from build123d import *

# Parameters (mm, degrees)
SKETCH1_W                  = 75
SKETCH1_H                  = 75
BOSS_EXTRUDE1_DEPTH        = 60
SKETCH2_R                  = 5
CUT_EXTRUDE1_DEPTH         = 20
FILLET1_R                  = 3
CUT_EXTRUDE2_DEPTH         = 5
FILLET2_R                  = 5
FILLET2_OF_MIRROR1_R       = 5
MIRROR2_START              = -7.071067908
MIRROR2_DEPTH              = 14.142135816
SKETCH4_W                  = 25
SKETCH4_H                  = 20
CUT_EXTRUDE3_DEPTH         = 55
FILLET3_R                  = 5
CUT_EXTRUDE4_DEPTH         = 81.078087059
CUT_EXTRUDE4_DEPTH_BACK    = 81.078087059
SKETCH5_R                  = 7.5
SKETCH7_R                  = 15
CUT_EXTRUDE5_DEPTH         = 15
SKETCH8_R                  = 4.5
CUT_EXTRUDE6_DEPTH         = 11
M5_TAPPED_HOLE1_AT_2_COUNT = 2
M5_TAPPED_HOLE1_AT_2_PITCH = 36
M8_TAPPED_HOLE1_D          = 6.8
M8_TAPPED_HOLE1_DEPTH      = 19.75
M8_TAPPED_HOLE1_TIP        = 2.042926105
F_8_0MM_DOWEL_HOLE1_D      = 8


# Read off the part's stored shape, not the designer's step: Mirror2
with BuildPart() as part:
    # Sketch1 → Boss-Extrude1 (new, symmetric)
    with BuildSketch(Plane.XY):
        Rectangle(SKETCH1_W, SKETCH1_H)
    extrude(amount=BOSS_EXTRUDE1_DEPTH, both=True)

    # Sketch2 → Cut-Extrude1 (cut)
    with BuildSketch(Plane(origin=(0, 37.5, 0), x_dir=(1, 0, 0), z_dir=(0, 1, 0))):
        with Locations(Location((0, 0, 0), (0, 0, 270))):
            Circle(SKETCH2_R)
    extrude(amount=-CUT_EXTRUDE1_DEPTH, mode=Mode.SUBTRACT)

    # Fillet1
    fillet1_edges = [part.edges().sort_by_distance(p)[0] for p in [
        (-37.5, 37.5, 0),
        (37.5, 37.5, 0),
    ]]
    fillet(fillet1_edges, radius=FILLET1_R)

    # Sketch3 → Cut-Extrude2 (cut, symmetric)
    with BuildSketch(Plane.XY.offset(-25)):
        Polygon((-37.5, 27.5), (-27.5, 37.5), (-37.5, 37.5), align=None)
    cut_extrude2 = extrude(amount=CUT_EXTRUDE2_DEPTH, both=True, mode=Mode.SUBTRACT)

    # Fillet2
    fillet2_edges = [part.edges().sort_by_distance(p)[0] for p in [
        (-32.5, 32.5, -30),
        (-32.5, 32.5, -20),
    ]]
    fillet(fillet2_edges, radius=FILLET2_R - 0.0001)  # a hair under: the kernel refuses the full size

    # Mirror1: Cut-Extrude2 across plane
    add(cut_extrude2.mirror(Plane.XY), mode=Mode.SUBTRACT)

    # Fillet2 of Mirror1
    fillet2_of_mirror1_edges = [part.edges().sort_by_distance(p)[0] for p in [
        (-32.5, 32.5, 30),
        (-32.5, 32.5, 20),
    ]]
    fillet(fillet2_of_mirror1_edges, radius=FILLET2_OF_MIRROR1_R - 0.0001)  # a hair under: the kernel refuses the full size

    # Mirror2 outline → Mirror2 (cut)
    with BuildSketch(Plane(origin=(0, 0, 0), x_dir=(0.707106781186546, 0.707106781186549, 0), z_dir=(0.707106781186549, -0.707106781186546, 0)).offset(MIRROR2_START)):
        with BuildLine():
            ThreePointArc((50.961940783, 30.000000002), (45.961940781, 25), (50.961940783, 19.999999998))
            Line((50.961940783, 19.999999998), (53, 20))
            Line((53, 20), (53, 30))
            Line((53, 30), (50.961940783, 30.000000002))
        make_face()
        with BuildLine():
            Line((53, -30), (53, -20))
            Line((53, -20), (50.961940783, -19.999999998))
            ThreePointArc((50.961940783, -19.999999998), (45.961940781, -25), (50.961940783, -30.000000002))
            Line((50.961940783, -30.000000002), (53, -30))
        make_face()
    extrude(amount=MIRROR2_DEPTH, mode=Mode.SUBTRACT)

    # Sketch4 → Cut-Extrude3 (cut)
    with BuildSketch(Plane.XZ.offset(37.5)):
        Rectangle(SKETCH4_W, SKETCH4_H)
    extrude(amount=-CUT_EXTRUDE3_DEPTH, mode=Mode.SUBTRACT)

    # Fillet3
    fillet3_edges = [part.edges().sort_by_distance(p)[0] for p in [
        (12.5, 17.5, 0),
        (12.5, -10, 10),
        (0, 17.5, -10),
        (12.5, -10, -10),
        (-12.5, 17.5, 0),
        (-12.5, -10, -10),
        (0, 17.5, 10),
        (-12.5, -10, 10),
    ]]
    fillet(fillet3_edges, radius=FILLET3_R - 0.0001)  # a hair under: the kernel refuses the full size

    # Sketch5 → Cut-Extrude4 (cut, two sides: drawn at the far end of the back side and taken through both)
    with BuildSketch(Plane(origin=(0, 0, 0), x_dir=(0, 0, -1), z_dir=(1, 0, 0)).offset(-CUT_EXTRUDE4_DEPTH_BACK)):
        with Locations((0, 7.5)):
            Circle(SKETCH5_R)
    extrude(amount=CUT_EXTRUDE4_DEPTH + CUT_EXTRUDE4_DEPTH_BACK, mode=Mode.SUBTRACT)

    # Sketch7 → Cut-Extrude5 (cut)
    with BuildSketch(Plane.ZY.offset(37.5)):
        with Locations((0, 7.5)):
            Circle(SKETCH7_R)
    cut_extrude5 = extrude(amount=-CUT_EXTRUDE5_DEPTH, mode=Mode.SUBTRACT)

    # Mirror3: Cut-Extrude5 across plane
    add(cut_extrude5.mirror(Plane(origin=(0, 0, 0), x_dir=(0, 0, 1), z_dir=(1, 0, 0))), mode=Mode.SUBTRACT)

    # Sketch8 → Cut-Extrude6 (cut)
    with BuildSketch(Plane.ZY.offset(37.5)):
        with Locations((-18, 7.5)):
            Circle(SKETCH8_R)
        with Locations((18, 7.5)):
            Circle(SKETCH8_R)
    cut_extrude6 = extrude(amount=-CUT_EXTRUDE6_DEPTH, mode=Mode.SUBTRACT)

    # Sketch10 → M5 Tapped Hole1 (revolve, cut)
    with BuildSketch(Plane(origin=(-26.5, 7.5, -18), x_dir=(0, 0, 1), z_dir=(0, 1, 0))):
        Polygon((0, 0), (0, 13.6618073), (2.1, 12.4), (2.1, 0), align=None)
    m5_tapped_hole1 = revolve(axis=Axis((-32.85, 7.5, -18), (1, 0, 0)), mode=Mode.SUBTRACT)

    # M5 Tapped Hole1 at 2: M5 Tapped Hole1 ×2
    with Locations(*[(0, 0, i * M5_TAPPED_HOLE1_AT_2_PITCH) for i in range(1, M5_TAPPED_HOLE1_AT_2_COUNT)]):
        add(m5_tapped_hole1, mode=Mode.SUBTRACT)

    # Mirror4: Cut-Extrude6, M5 Tapped Hole1 across plane
    add(cut_extrude6.mirror(Plane(origin=(0, 0, 0), x_dir=(0, 0, 1), z_dir=(1, 0, 0))), mode=Mode.SUBTRACT)
    add(m5_tapped_hole1.mirror(Plane(origin=(0, 0, 0), x_dir=(0, 0, 1), z_dir=(1, 0, 0))), mode=Mode.SUBTRACT)

    # Mirror4 copy 1 sketch → Mirror4 copy 1 (revolve, cut)
    with BuildSketch(Plane(origin=(26.5, 7.5, 18), x_dir=(0, 0, 1), z_dir=(0, 1, 0))):
        Polygon((0, 0), (0, -13.6618073), (2.1, -12.4), (2.1, 0), align=None)
    revolve(axis=Axis((32.85, 7.5, 18), (1, 0, 0)), mode=Mode.SUBTRACT)

    # M8 Tapped Hole1
    with Locations(Plane(origin=(0, -37.5, 0), x_dir=(-1, 0, 0), z_dir=(0, -1, 0))):
        with Locations((-25.5, 48), (25.5, 48), (25.5, -48), (-25.5, -48)):
            Hole(M8_TAPPED_HOLE1_D / 2, depth=M8_TAPPED_HOLE1_DEPTH)
            with Locations((0, 0, -(M8_TAPPED_HOLE1_DEPTH + M8_TAPPED_HOLE1_TIP / 2))):  # 118° drill point
                Cone(0, M8_TAPPED_HOLE1_D / 2, M8_TAPPED_HOLE1_TIP, mode=Mode.SUBTRACT)

    # Ø8.0mm Dowel Hole1 (through all)
    with Locations(Plane(origin=(0, -37.5, 0), x_dir=(-1, 0, 0), z_dir=(0, -1, 0))):
        with Locations((0, 48), (0, -48)):
            Hole(F_8_0MM_DOWEL_HOLE1_D / 2)


solid = part.part
Input: part model. Units: mm. Frame: model coordinates. A direction names the side the tool comes from. Coordinates: 2 decimals unless noted, no trailing zeros. Loops run counter-clockwise (first coordinate to the right, second up) from the corner with the lowest first, then second, coordinate; pieces in that order, holes last. Notation, with made-up numbers: (11.5, 52.5) - (28.5, 52.5) arc R12 cw to (28.5, 63.5) - close; hole circle Ø6 at (85.25, 86.25). An arc over 180 degrees is marked (long way). Answer in a Markdown table with one row per item. Add a question column.
Item 1: Line query: line 1 along X through (y, z) = (-21, -48); line 2 along Z through (x, y) = (-25.5, -25.75); line 3 along Z through (x, y) = (35, 7). Output: solid intervals per line, ascending. Write a range as [from, to].
Item 2: Section query C-C on y = -11. Return the cut outline in (x, z).
Item 3: Contact query for flat-ended pins moving along their axis: P1, Ø18, axis at y = 7.5, z = 0, coming from the -X side; P2, Ø7, axis at y = 7.5, z = -18, coming from the -X side; P3, Ø5.5, axis at x = -25.5, z = 48, coming from the -Y side. Output: stop coordinate, or through.
Item 4: Mould query, pull axis Z, two halves, no side actions, for faces 5 (the conical face through (25.628, -16.062, -47.424)), 6 (the cylindrical face through (36.6, 36.64, 44.79)). Classes: released by +Z, released by -Z, zero draft, split by the parting line, or undercut.
Item 5: Access query for faces 1 (the cylindrical face through (-10.219, 16.696, 0.07)), 2 (the flat face through (36.2, 36.3, -20)), 3 (the flat face through (-26.5, 7.6, 20.3)), 4 (the cylindrical face through (20.39, 5.73, -16.87)). Directions: +Z, -Z, +X, -X, +Y, -Y. A direction counts if a zero-diameter tool reaches every point of the face in a straight line with its end or side. Return the directions, or none.
Item 6: Section query A-A on z = 0. State how many separate pieces and enclosed holes the cut face has, then the cut area to 3 significant figures.
Item 7: Section query B-B on y = -23. Return the cut outline in (x, z), then the cut area to 3 significant figures.
Recorded:
| question | item | result |
|---|---|---|
| 1 | line 1 | [-37.5, -28.9], [-22.1, -4], [4, 22.1], [28.9, 37.5] |
| 1 | line 2 | [-60, -51.4], [-44.6, 44.6], [51.4, 60] |
| 1 | line 3 | [-60, -22.47], [22.47, 60] |
| 2 | outline | (-37.5, -60) - (37.5, -60) - (37.5, 60) - (-37.5, 60) - close; hole (-12.5, -5) arc R5 ccw to (-7.5, -10) - (7.5, -10) arc R5 ccw to (12.5, -5) - (12.5, 5) arc R5 ccw to (7.5, 10) - (-7.5, 10) arc R5 ccw to (-12.5, 5) - close; hole circle Ø8 at (0, -48); hole circle Ø8 at (0, 48) |
| 3 | P1 | x = -22.5 |
| 3 | P2 | x = -26.5 |
| 3 | P3 | y = -17.36 |
| 4 | face 5 | undercut |
| 4 | face 6 | zero draft |
| 5 | face 1 | -Y |
| 5 | face 2 | +X, +Y |
| 5 | face 3 | -X |
| 5 | face 4 | +X |
| 6 | separate pieces | 4 |
| 6 | enclosed holes | 0 |
| 6 | area | 2,860 mm^2 |
| 7 | outline | (-37.5, -60) - (37.5, -60) - (37.5, 60) - (-37.5, 60) - close; hole circle Ø6.8 at (-25.5, -48); hole circle Ø6.8 at (-25.5, 48); hole (-12.5, -5) arc R5 ccw to (-7.5, -10) - (7.5, -10) arc R5 ccw to (12.5, -5) - (12.5, 5) arc R5 ccw to (7.5, 10) - (-7.5, 10) arc R5 ccw to (-12.5, 5) - close; hole circle Ø8 at (0, -48); hole circle Ø8 at (0, 48); hole circle Ø6.8 at (25.5, -48); hole circle Ø6.8 at (25.5, 48) |
| 7 | area | 8,280 mm^2 |
